Job drawing, mm, ordinate dimensions from the low corner. One solid piece. A direction names the side the tool comes from. Round coordinates to 2 decimals unless told otherwise and drop trailing zeros. Loops run counter-clockwise (first coordinate to the right, second up) from the corner with the lowest first, then second, coordinate; pieces in that order, holes last. Notation, with made-up numbers: (15.25, 48) - (74.25, 48) arc R20 ccw to (74.25, 70) - close; hole circle Ø9 at (15.5, -11.5). An arc over 180 degrees is marked (long way). One line per question, with ' | ' between items. Start each with the question number.
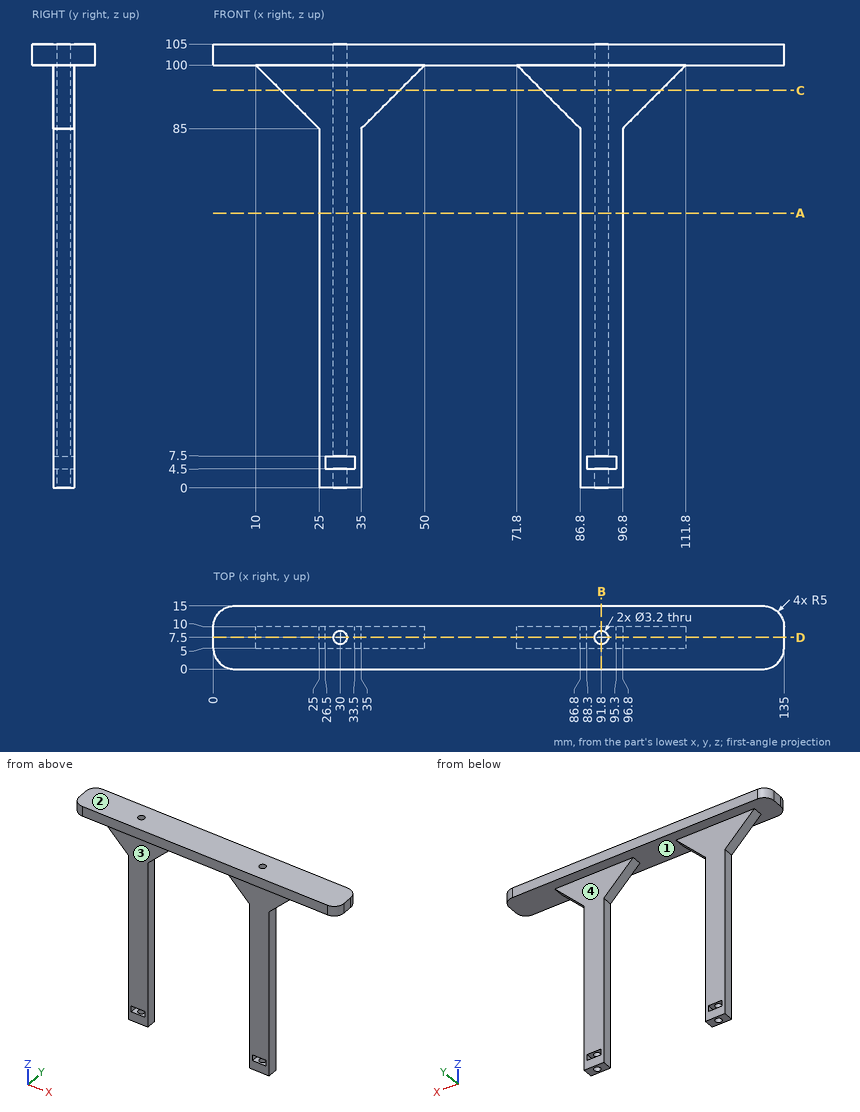
1) Saw through at A-A on z = 65. Write the cut outline in (x, y).
2) Tool access for the marked faces 1, 2, 3 and 4: list every direction of +Z, -Z, +X, -X, +Y, -Y with a clear straight run to the whole face (end or side of a thin tool).
3) Saw through at B-B on x = 91.8. Write the cut outline in (y, z).
4) Saw through at C-C on z = 94. Write the cut outline in (x, y), and give its area (3 significant figures).
5) Wall check: line 1 (X direction, y = 7.75, z = 71); line 2 (X direction, y = 9.5, z = 28.5); line 3 (Z direction, x = 56, y = 9.5). Give the ranges that are in metal, low to high. Write a range as [from, to].
6) Saw through at D-D on y = 7.5. State how many separate pieces and enclosed holes the cut face has, and give its area (3 significant figures).
7) Drop flat-ended pins along their axis: pin 1 (2.5 mm diameter, centred on y = 8.5, z = 39.5, fed in from -X); pin 2 (8 mm diameter, centred on x = 86.5, z = 14.5, fed in from +Y); pin 3 (3.5 mm diameter, centred on y = 8, z = 5.5, fed in from +X); pin 4 (5 mm diameter, centred on x = 100.5, z = 57, fed in from -Y). Give the stop position or say it passes through.
Answer key:
1) outline: (25, 5) - (35, 5) - (35, 10) - (25, 10) - close; (86.8, 5) - (96.8, 5) - (96.8, 10) - (86.8, 10) - close; hole circle Ø3.2 at (30, 7.5); hole circle Ø3.2 at (91.8, 7.5)
2) face 1: -Z | face 2: +Z, +X, -X, +Y, -Y | face 3: -Z, +X, -X, -Y | face 4: -Z, +X, -X, +Y
3) outline: (0, 100) - (5, 100) - (5, 7.5) - (5.9, 7.5) - (5.9, 105) - (0, 105) - close; (5, 0) - (5.9, 0) - (5.9, 4.5) - (5, 4.5) - close; (9.1, 0) - (10, 0) - (10, 4.5) - (9.1, 4.5) - close; (9.1, 7.5) - (10, 7.5) - (10, 100) - (15, 100) - (15, 105) - (9.1, 105) - close
4) outline: (16, 5) - (44, 5) - (44, 10) - (16, 10) - close; (77.8, 5) - (105.8, 5) - (105.8, 10) - (77.8, 10) - close; hole circle Ø3.2 at (30, 7.5); hole circle Ø3.2 at (91.8, 7.5) | area: 264 mm²
5) line 1: [25, 28.42], [31.58, 35], [86.8, 90.22], [93.38, 96.8] | line 2: [25, 35], [86.8, 96.8] | line 3: [100, 105]
6) separate pieces: 3 | enclosed holes: 0 | area: 2,430 mm²
7) pin 1: x = 25 | pin 2: y = 10 | pin 3: x = 96.8 | pin 4: through
